Drawing for the job (mm, zero at the part's lowest x, y, z). A direction names the side the tool comes from. Give positions to 0.01 mm unless a question says otherwise; leave off trailing zeros. Order: outer loops, then holes, each group sorted by start corner. A loop starts at its lowest first (then second) coordinate and runs counter-clockwise, first axis right, second up. Notation, with made-up numbers: (69, 31.5) -> (123, 31.5) arc R22 cw to (123, 51.5) -> close; hole circle Ø10 at (26.5, -34). An arc over 180 degrees is marked (long way). Use one line per item in the form item = value. Start each with the question number.
1) Cut at B-B, the plane z = 40. Give the cut face in (x, y).
2) Drop flat-ended pins along their axis: P1, Ø12, axis at y = 53.5, z = 47.5, coming from the -X side; P2, Ø8, axis at x = 14.5, z = 22.5, coming from the +Y side. Give the stop position or say it passes through.
3) Tool access for the marked faces 1 and 2: list every direction of +Z, -Z, +X, -X, +Y, -Y with a clear straight run to the whole face (end or side of a thin tool).
4) Cut at A-A, the plane x = 40. Give the cut face in (y, z).
5) Cut at C-C, the plane y = 70. Give the cut face in (x, z).
6) Probe line 1 (Z direction, x = 40, y = 1.2); line 2 (Y direction, x = 69.5, z = 52); line 3 (X direction, y = 122, z = 33). List the from-to ranges inside material, lowest first.
7) Cut at D-D, the plane z = 58.5. Give the cut face in (x, y) (1 decimal).
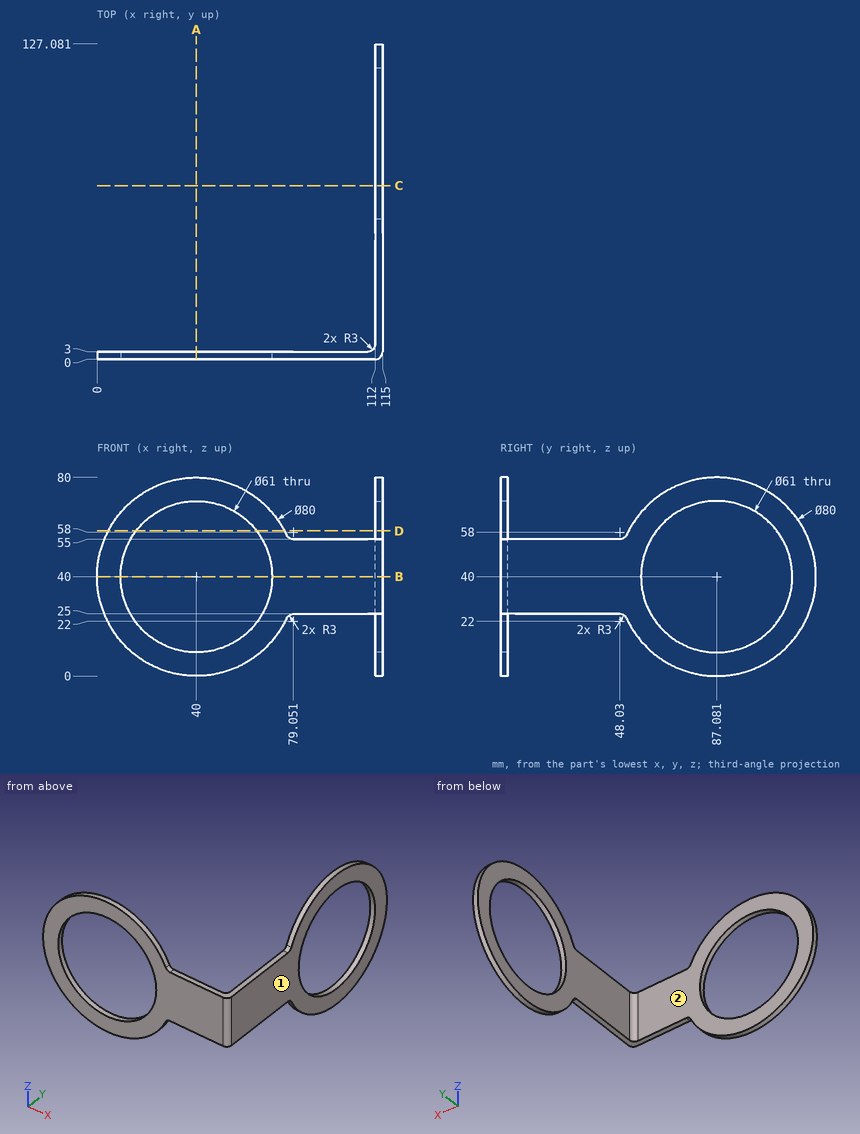
Result:
q1.outline = (0, 0) -> (9.5, 0) -> (9.5, 3) -> (0, 3) -> close; (70.5, 0) -> (112, 0) arc R3 ccw to (115, 3) -> (115, 56.58) -> (112, 56.58) -> (112, 6) arc R3 cw to (109, 3) -> (70.5, 3) -> close; (112, 117.58) -> (115, 117.58) -> (115, 127.08) -> (112, 127.08) -> close
q2.P1 = 112
q2.P2 = 3
q3.face_1 = +Z, -Z, +X, +Y, -Y
q3.face_2 = +Z, -Z, -X, +Y
q4.outline = (0, 0) -> (3, 0) -> (3, 9.5) -> (0, 9.5) -> close; (0, 70.5) -> (3, 70.5) -> (3, 80) -> (0, 80) -> close
q5.outline = (112, 3.83) -> (115, 3.83) -> (115, 14.73) -> (112, 14.73) -> close; (112, 65.27) -> (115, 65.27) -> (115, 76.17) -> (112, 76.17) -> close
q6.line_1 = 0 to 9.5, 70.5 to 80
q6.line_2 = 0 to 3
q6.line_3 = 112 to 115
q7.outline = (4.5, 0) -> (15.8, 0) -> (15.8, 3) -> (4.5, 3) -> close; (64.2, 0) -> (75.5, 0) -> (75.5, 3) -> (64.2, 3) -> close; (112, 51.6) -> (115, 51.6) -> (115, 62.8) -> (112, 62.8) -> close; (112, 111.3) -> (115, 111.3) -> (115, 122.5) -> (112, 122.5) -> close
